from build123d import *

# Parameters (mm, degrees)
SKETCH1_R           = 53.594
SKETCH1_R_2         = 51.054
BOSS_EXTRUDE2_DEPTH = 6.35
BOSS_EXTRUDE3_START = 2.54
SKETCH2_R           = 53.594
BOSS_EXTRUDE3_DEPTH = 2.54
SKETCH4_W           = 25.4
SKETCH4_H           = 2.794
CUT_EXTRUDE1_DEPTH  = 77.058899361
CUT_EXTRUDE2_DEPTH  = 77.312946294


with BuildPart() as part:
    # Sketch1 → Boss-Extrude2 (new body)
    with BuildSketch(Plane(origin=(0, 0, 0), x_dir=(1, 0, 0), z_dir=(0, 1, 0))):
        with Locations(Location((0, 0, 0), (0, 0, 270))):
            Circle(SKETCH1_R)
        with Locations(Location((0, 0, 0), (0, 0, 270))):
            Circle(SKETCH1_R_2, mode=Mode.SUBTRACT)
    extrude(amount=BOSS_EXTRUDE2_DEPTH)

    # Sketch2 → Boss-Extrude3 (add)
    with BuildSketch(Plane.XZ.offset(BOSS_EXTRUDE3_START)):
        with Locations(Location((0, 0, 0), (0, 0, 270))):
            Circle(SKETCH2_R)
    extrude(amount=-BOSS_EXTRUDE3_DEPTH)

    # Sketch4 → Cut-Extrude1 (cut, through all)
    with BuildSketch(Plane(origin=(0, 0, 0), x_dir=(1, 0, 0), z_dir=(0, 1, 0))):
        with Locations((-25.4, 19.05)):
            Rectangle(SKETCH4_W, SKETCH4_H)
        with Locations((25.4, 19.05)):
            Rectangle(SKETCH4_W, SKETCH4_H)
    extrude(amount=-CUT_EXTRUDE1_DEPTH, mode=Mode.SUBTRACT)

    # Sketch5 → Cut-Extrude2 (cut, through all)
    with BuildSketch(Plane.XZ.offset(2.54)):
        Polygon((-349.002283825, 0), (-69.85, 0), (69.85, 0), (349.002283825, 0), (349.002283825, 558.304567649), (-349.002283825, 558.304567649), align=None)
    extrude(amount=-CUT_EXTRUDE2_DEPTH, mode=Mode.SUBTRACT)


solid = part.part
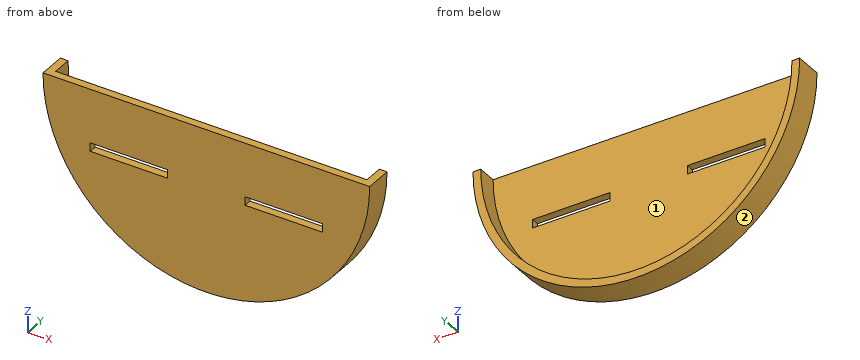
Geometry: final body of the model. Coordinates: model frame, mm. Face numbers are marked on the shaded views. A direction names the side the tool comes from. Coordinates: 2 decimals unless noted, no trailing zeros. Loops run counter-clockwise (first coordinate to the right, second up) from the corner with the lowest first, then second, coordinate; pieces in that order, holes last. Notation, with made-up numbers: (76.25, 78.25) - (117.25, 78.25) arc R25 ccw to (117.25, 91.25) - close; hole circle Ø11 at (68, 71.25). An arc over 180 degrees is marked (long way). One line per question, with ' | ' between items. Start each with the question number.
(1) Cut plane B-B on x = 0. Output: boundary loops of the cut face in (y, z).
(2) Cut plane C-C on z = -14. Output: boundary loops of the cut face in (x, y).
(3) First-contact query: pin 1 (0.8 mm diameter, centred on y = -1.5, z = -19.5, fed in from +X) (3 decimals); pin 2 (2 mm diameter, centred on x = 24, y = -1, fed in from -Z); pin 3 (1 mm diameter, centred on x = -26, z = -42.5, fed in from +Y). Flat tips, straight axial feed; report the tip coordinate or a pass-through.
(4) Cut plane D-D on y = 5. Output: boundary loops of the cut face in (x, z), and give its area (3 significant figures).
(5) Reachability of the marked faces 1 and 2 from +Z, -Z, +X, -X, +Y, -Y: full face, straight path, thin tool, end or side. Return the list, or none.
(6) Cut plane A-A on x = 32. Output: boundary loops of the cut face in (y, z), and give its area (3 significant figures).
(7) Ray query, L1, parallel to Z at x = 0.5, y = 0.25; L2, parallel to Y at x = -26, z = -25; L3, parallel to Z at x = -27.5, y = -0.5. Return the intervals inside material, ascending. Write a range as from..to.
Here are the results:
1) outline: (-2.54, -53.59) - (6.35, -53.59) - (6.35, -51.05) - (0, -51.05) - (0, 0) - (-2.54, 0) - close
2) outline: (-51.73, -2.54) - (51.73, -2.54) - (51.73, 6.35) - (49.1, 6.35) - (49.1, 0) - (-49.1, 0) - (-49.1, 6.35) - (-51.73, 6.35) - close
3) pin 1: x = 50.075 | pin 2: z = -48.41 | pin 3: y = 0
4) outline: (-53.59, 0) arc R53.59 ccw to (53.59, 0) - (51.05, 0) arc R51.05 cw to (-51.05, 0) - close | area: 418 mm²
5) face 1: +Z, +Y | face 2: -Z, +Y, -Y
6) outline: (-2.54, -42.99) - (6.35, -42.99) - (6.35, -39.78) - (0, -39.78) - (0, -20.45) - (-2.54, -20.45) - close; (-2.54, -17.65) - (0, -17.65) - (0, 0) - (-2.54, 0) - close | area: 122 mm²
7) L1: -53.59..-51.05 | L2: -2.54..0 | L3: -46..-20.45, -17.65..0
